Source: CAD feature listing. Evaluate the final solid. Frame: model axes, mm. A direction names the side the tool comes from. Coordinates: 2 decimals unless noted, no trailing zeros. Order: outer loops, then holes, each group sorted by start corner. A loop starts at its lowest first (then second) coordinate and runs counter-clockwise, first axis right, second up. Notation, with made-up numbers: (8.5, -39) - (29.5, -39) arc R9 ccw to (29.5, -28) - close; hole circle Ø3 at (24.25, 9). An arc over 180 degrees is marked (long way). One line per question, with ' | ' between items. Start each with the question number.
(1) Section C-C (y = 9). Return the cut outline in (x, z).
(2) Section B-B (z = -55.5). Return the cut outline in (x, y).
(3) Section A-A (x = 2.2). Return the cut outline in (y, z), then the cut area to 3 significant figures.
(4) Contact query for a flat-ended pin moving along its axis: P1, Ø1.2, axis at x = 2, y = 8, coming from the -Z side. Output: stop coordinate, or through.
(5) Draft query along Z for faces 3 (the flat face through (2, 26, -25)), 4 (the flat face through (2, 13, -60)), 5 (the flat face through (2, 11, -4)). Return one class per face: +Z half, -Z half, draft (parallel to the pull), parting line (faces both ways), or undercut.
(6) Section D-D (y = 23.75). Return the cut outline in (x, z).
(7) Line query: line 1 along Y through (x, z) = (0.5, -20); line 2 along Z through (x, y) = (2.55, 13); line 3 along Y through (x, z) = (0.65, -59.5). Output: solid intervals per line, ascending.
(8) Access query for faces 1 (the flat face through (2, 0, -35)), 2 (the flat face through (2, 11, 0)). Directions: +Z, -Z, +X, -X, +Y, -Y. A direction counts if a zero-diameter tool reaches every point of the face in a straight line with its end or side. Return the directions, or none.
Autodesk Inventor part; units mm, degrees
ref_plane "YZ Plane" through (0, 0, 0) normal (1, 0, 0) x (0, 1, 0)
ref_plane "XZ Plane" through (0, 0, 0) normal (0, 1, 0) x (-1, 0, 0)
ref_plane "XY Plane" through (0, 0, 0) normal (0, 0, 1) x (1, 0, 0)
sketch "Sketch1" plane through (0, 0, 0) normal (1, 0, 0) x (0, 1, 0)
  line L0 (0, 0) -> (-4, 0)
  line L1 (-4, 0) -> (-4, -70)
  line L2 (-4, -70) -> (0, -70)
  line L3 (0, -70) -> (0, -4)
  line L4 (-4, 0) -> (26, 0)
  line L5 (26, 0) -> (26, -4)
  line L6 (22, -4) -> (0, -4)
  line L7 (-4, -4) -> (-4, 0)
  line L8 (26, 0) -> (22, 0)
  line L9 (22, -4) -> (22, -50)
  line L10 (22, -50) -> (26, -50)
  line L11 (26, -50) -> (26, 0)
  line L12 (26, -50) -> (0, -70)
  line L13 (0, -70) -> (0, -66)
  line L14 (0, -66) -> (22, -49.2125)
  dimension "d0" = 4
  dimension "d1" = 70
  dimension "d2" = 30
  dimension "d3" = 4
  dimension "d4" = 4
  dimension "d5" = 50
  dimension "d6" = 4
extrude "Extrusion1" add sketch "Sketch1" along normal blind 4 contours L4 L5 L11 L10 L9 L6 L3 L2 L1 L0 | L3 L14 L9 L10 L12
properties part number "Holder Motor Lifter_3DPrint"
Response values:
1) outline: (0, -63.08) - (4, -63.08) - (4, -59.13) - (0, -59.13) - close; (0, -4) - (4, -4) - (4, 0) - (0, 0) - close
2) outline: (0, -4) - (4, -4) - (4, 0) - (0, 0) - close; (0, 13.76) - (4, 13.76) - (4, 18.85) - (0, 18.85) - close
3) outline: (-4, -70) - (0, -70) - (26, -50) - (26, 0) - (-4, 0) - close; hole (0, -66) - (22, -49.21) - (22, -4) - (0, -4) - close | area: 661 mm²
4) P1: stops at z = -64.31
5) face 3: draft | face 4: -Z half | face 5: undercut
6) outline: (0, -51.73) - (4, -51.73) - (4, 0) - (0, 0) - close
7) line 1: y = -4 to 0, 22 to 26 | line 2: z = -60 to -56.08, -4 to 0 | line 3: y = -4 to 0, 8.52 to 13.65
8) face 1: +X, -X | face 2: +Z, +X, -X, +Y, -Y
